from build123d import *

# Parameters (mm, degrees)
SKETCH2_W           = 147.32
SKETCH2_H           = 104.648
BOSS_EXTRUDE1_DEPTH = 5.08
SKETCH3_R           = 19.05
CUT_EXTRUDE1_DEPTH  = 2.54
SKETCH4_R           = 12.7
CUT_EXTRUDE2_DEPTH  = 3.81
SKETCH5_W           = 6.35
SKETCH5_H           = 6.35
CUT_EXTRUDE3_DEPTH  = 6.35


with BuildPart() as part:
    # Sketch2 → Boss-Extrude1 (new body)
    with BuildSketch(Plane.XY):
        with Locations((117.825395055, 78.266401141)):
            Rectangle(SKETCH2_W, SKETCH2_H)
    extrude(amount=BOSS_EXTRUDE1_DEPTH)

    # Sketch3 → Cut-Extrude1 (cut)
    with BuildSketch(Plane.XY):
        with Locations((69.599550134, 110.562048191)):
            Circle(SKETCH3_R)
        with Locations((69.599550134, 45.622553044)):
            Circle(SKETCH3_R)
        with Locations((92.580819194, 77.831149833)):
            Circle(SKETCH3_R)
        with Locations((115.562088254, 110.562048191)):
            Circle(SKETCH3_R)
        with Locations((115.562088254, 45.622553044)):
            Circle(SKETCH3_R)
        with Locations((140.284362546, 77.831149833)):
            Circle(SKETCH3_R)
        with Locations((165.877139454, 110.562048191)):
            Circle(SKETCH3_R)
        with Locations((165.877139454, 45.622553044)):
            Circle(SKETCH3_R)
    extrude(amount=CUT_EXTRUDE1_DEPTH, mode=Mode.SUBTRACT)

    # Sketch4 → Cut-Extrude2 (cut)
    with BuildSketch(Plane.XY):
        with Locations((69.599550134, 45.622553044)):
            Circle(SKETCH4_R)
        with Locations((115.562088254, 45.622553044)):
            Circle(SKETCH4_R)
        with Locations((165.877139454, 45.622553044)):
            Circle(SKETCH4_R)
        with Locations((92.580819194, 77.831149833)):
            Circle(SKETCH4_R)
        with Locations((140.284362546, 77.831149833)):
            Circle(SKETCH4_R)
        with Locations((69.599550134, 110.562048191)):
            Circle(SKETCH4_R)
        with Locations((115.562088254, 110.562048191)):
            Circle(SKETCH4_R)
        with Locations((165.877139454, 110.562048191)):
            Circle(SKETCH4_R)
    extrude(amount=CUT_EXTRUDE2_DEPTH, mode=Mode.SUBTRACT)

    # Sketch5 → Cut-Extrude3 (cut)
    with BuildSketch(Plane.XY):
        with Locations((48.615350013, 29.461567224)):
            Rectangle(SKETCH5_W, SKETCH5_H)
        with Locations((186.994201874, 29.461567224)):
            Rectangle(SKETCH5_W, SKETCH5_H)
        with Locations((186.994201874, 126.386007845)):
            Rectangle(SKETCH5_W, SKETCH5_H)
        with Locations((48.615350013, 126.386007845)):
            Rectangle(SKETCH5_W, SKETCH5_H)
    extrude(amount=CUT_EXTRUDE3_DEPTH, mode=Mode.SUBTRACT)


solid = part.part
Here's how the part is built. I have some questions about the finished solid (model axes, mm). A direction names the side the tool comes from. Coordinates: 2 decimals unless noted, no trailing zeros. Order: outer loops, then holes, each group sorted by start corner. A loop starts at its lowest first (then second) coordinate and runs counter-clockwise, first axis right, second up. Notation, with made-up numbers: (44.25, 48.25) -> (63.25, 48.25) arc R23 ccw to (63.25, 74.25) -> close; hole circle Ø7 at (9, -37). An arc over 180 degrees is marked (long way). Answer in a Markdown table with one row per item.
(1) On a 3-axis mill with a long thin cutter (end or side, diameter ignored), from which of +Z, -Z, +X, -X, +Y, -Y can I reach the whole of each face in a straight line? I mean faces 1 (the face through (104.694, 81.646, 3.166)), 2 (the face through (51.79, 29, 3)). Say none if no direction works.
Answer key:
| item | result |
|---|---|
| face 1 | -Z |
| face 2 | +Z, -Z |
(2) I want a section at D-D on y = 94.5. List the corners of the cut face in (x, z) for me.
Answer key:
| item | result |
|---|---|
| outline | (44.17, 0) -> (59.36, 0) -> (59.36, 2.54) -> (79.84, 2.54) -> (79.84, 0) -> (83.36, 0) -> (83.36, 2.54) -> (101.8, 2.54) -> (101.8, 0) -> (105.32, 0) -> (105.32, 2.54) -> (125.8, 2.54) -> (125.8, 0) -> (131.06, 0) -> (131.06, 2.54) -> (149.51, 2.54) -> (149.51, 0) -> (155.63, 0) -> (155.63, 2.54) -> (176.12, 2.54) -> (176.12, 0) -> (191.49, 0) -> (191.49, 5.08) -> (44.17, 5.08) -> close |
(3) Thinking about a two-plate mould opening in X: for faces 3 (the face through (117, 79, 5.08)), 4 (the face through (81.71, 114.38, 3.17)), which applies, +X half, -X half, draft (parallel to the pull), parting line (faces both ways), or undercut?
Answer key:
| item | result |
|---|---|
| face 3 | draft |
| face 4 | undercut |
(4) Will this pin go through, and if not, where does the flat tip stop? pin 1 Ø12.5 at (x, y) = (73, 41) entering from -Z.
Answer key:
| item | result |
|---|---|
| pin 1 | z = 3.81 |
(5) I want a section at C-C on x = 76.5. List the corners of the cut face in (y, z) for me, then the cut area to 3 significant figures.
Answer key:
| item | result |
|---|---|
| outline | (25.94, 0) -> (27.87, 0) -> (27.87, 2.54) -> (34.96, 2.54) -> (34.96, 3.81) -> (56.28, 3.81) -> (56.28, 2.54) -> (63.38, 2.54) -> (63.38, 0) -> (67.62, 0) -> (67.62, 2.54) -> (88.04, 2.54) -> (88.04, 0) -> (92.81, 0) -> (92.81, 2.54) -> (99.9, 2.54) -> (99.9, 3.81) -> (121.22, 3.81) -> (121.22, 2.54) -> (128.32, 2.54) -> (128.32, 0) -> (130.59, 0) -> (130.59, 5.08) -> (25.94, 5.08) -> close |
| area | 245 mm^2 |
(6) Please list where these lines run through material, in increasing order: probe 1 along Y at (x, z) = (50, 4.7); probe 2 along X at (y, z) = (125.5, 3.2); probe 3 along X at (y, z) = (57, 1.65).
Answer key:
| item | result |
|---|---|
| probe 1 | 25.94 to 26.29, 32.64 to 123.21, 129.56 to 130.59 |
| probe 2 | 44.17 to 45.44, 51.79 to 183.82, 190.17 to 191.49 |
| probe 3 | 44.17 to 54.32, 84.88 to 100.28, 130.84 to 150.6, 181.16 to 191.49 |
(7) I want a section at B-B on y = 114. List the corners of the cut face in (x, z) for me.
Answer key:
| item | result |
|---|---|
| outline | (44.17, 0) -> (50.86, 0) -> (50.86, 2.54) -> (57.37, 2.54) -> (57.37, 3.81) -> (81.83, 3.81) -> (81.83, 2.54) -> (88.34, 2.54) -> (88.34, 0) -> (96.82, 0) -> (96.82, 2.54) -> (103.34, 2.54) -> (103.34, 3.81) -> (127.79, 3.81) -> (127.79, 2.54) -> (134.3, 2.54) -> (134.3, 0) -> (147.14, 0) -> (147.14, 2.54) -> (153.65, 2.54) -> (153.65, 3.81) -> (178.1, 3.81) -> (178.1, 2.54) -> (184.61, 2.54) -> (184.61, 0) -> (191.49, 0) -> (191.49, 5.08) -> (44.17, 5.08) -> close |
(8) I want a section at A-A on z = 0.9. Count the separate pieces of the cut face and the enclosed holes in it, then the cut area to 3 significant figures.
Answer key:
| item | result |
|---|---|
| separate pieces | 1 |
| enclosed holes | 12 |
| area | 6,130 mm^2 |
